Build history of the part. All positions in model axes, mm. A direction names the side the tool comes from. Round coordinates to 2 decimals unless told otherwise and drop trailing zeros. Write each loop counter-clockwise with the first axis right and the second up, starting at its lowest first coordinate (ties: lowest second). Pieces come first, ordered by that corner, then holes.
Item 1: 3-axis set-ups, long thin cutter, end or side, ignore diameter. For faces 1 (the flat face through (4.261, -19, 3)), 2 (the cylindrical face through (-3.69, -30.38, 2.46)): which of +Z, -Z, +X, -X, +Y, -Y reach the whole face in a straight line?
Item 2: Band-saw the part on D-D, the plane y = -27.5. Write the cut outline in (x, z), then the cut area to 3 significant figures.
Item 3: Drop flat-ended pins along their axis: pin 1 Ø2 at (y, z) = (-8.5, 2.5) entering from +X; pin 2 Ø1.5 at (x, z) = (5.5, 1.5) entering from -Y; pin 3 Ø2 at (y, z) = (-12.5, 1) entering from -X. Give the stop position or say it passes through.
Item 4: Band-saw the part on B-B, the plane y = 0. Write the cut outline in (x, z), then the cut area to 3 significant figures.
Item 5: Band-saw the part on A-A, the plane x = 0. Write the cut outline in (y, z), then the cut area to 3 significant figures.
Item 6: Mould opens along X. For faces 3 (the flat face through (0, -6, 5)), 4 (the cylindrical face through (-3, 0, 2)), 5 (the flat face through (-4.261, -19, 3)) say: +X half, -X half, draft (parallel to the pull), parting line (faces both ways), or undercut.
Item 7: Band-saw the part on C-C, the plane z = 1.6. Write the cut outline in (x, y), then the cut area to 3 significant figures.
Item 8: Wall check: probe 1 along Y at (x, z) = (0, 3.8); probe 2 along Y at (x, z) = (1.25, 1.45); probe 3 along X at (y, z) = (-22.5, 3.25). Give the ranges that are in metal, low to high.
```python
from build123d import *

# Parameters (mm, degrees)
F0_R     = 10
F0_R_2   = 3
F1_DEPTH = 5
F3_DEPTH = 5
F4_R     = 2
F5_R     = 2
F6_DEPTH = 5.001


with BuildPart() as f1:
    # F0 (on Top) → F1 (new body)
    with BuildSketch(Plane.XY):
        Circle(F0_R)
        Circle(F0_R_2, mode=Mode.SUBTRACT)
    extrude(amount=F1_DEPTH)

    # F2 (on face) → F3 (join)
    with BuildSketch(Plane.XY.offset(5)):
        with BuildLine():
            Line((4.2607685338, -30.9823937714), (4.2607685338, -9.0468697073))
            ThreePointArc((4.2607685338, -9.0468697073), (0, -10), (-4.2607685338, -9.0468697073))
            Line((-4.2607685338, -9.0468697073), (-4.2607685338, -30.9823937714))
            Line((-4.2607685338, -30.9823937714), (4.2607685338, -30.9823937714))
        make_face()
    extrude(amount=-F3_DEPTH)

    # F4
    f4_edges = [f1.edges().sort_by_distance(p)[0] for p in [
        (-4.260769, -30.982394, 2.5),
        (4.260769, -30.982394, 2.5),
    ]]
    fillet(f4_edges, radius=F4_R)

    # F5 (on face) → F6 (cut, through all)
    with BuildSketch(Plane.XY.offset(5)):
        with Locations((0, -26.1633973569)):
            Circle(F5_R)
    extrude(amount=-F6_DEPTH, mode=Mode.SUBTRACT)


solid = f1.part
```
Results:
1. face 1: +Z, -Z, +X, -Y
1. face 2: +Z, -Z, -X, -Y
2. outline: (-4.26, 0) - (-1.49, 0) - (-1.49, 5) - (-4.26, 5) - close; (1.49, 0) - (4.26, 0) - (4.26, 5) - (1.49, 5) - close
2. area: 27.7 mm2
3. pin 1: stops at x = 6.61
3. pin 2: stops at y = -8.8
3. pin 3: stops at x = -4.26
4. outline: (-10, 0) - (-3, 0) - (-3, 5) - (-10, 5) - close; (3, 0) - (10, 0) - (10, 5) - (3, 5) - close
4. area: 70.0 mm2
5. outline: (-30.98, 0) - (-28.16, 0) - (-28.16, 5) - (-30.98, 5) - close; (-24.16, 0) - (-3, 0) - (-3, 5) - (-24.16, 5) - close; (3, 0) - (10, 0) - (10, 5) - (3, 5) - close
5. area: 155 mm2
6. face 3: draft
6. face 4: undercut
6. face 5: -X half
7. outline: (-4.26, -28.98) arc R2 ccw to (-2.26, -30.98) - (2.26, -30.98) arc R2 ccw to (4.26, -28.98) - (4.26, -9.05) arc R10 ccw (long way) to (-4.26, -9.05) - close; hole circle Ø6 at (0, 0); hole circle Ø4 at (0, -26.16)
7. area: 453 mm2
8. probe 1: y = -30.98 to -28.16, -24.16 to -3, 3 to 10
8. probe 2: y = -30.98 to -27.72, -24.6 to -2.73, 2.73 to 9.92
8. probe 3: x = -4.26 to 4.26
